The drawing under review shows one solid part. Ordinate dimensions are in mm from its lowest x, y, z. A direction names the side the tool comes from. Coordinates: 2 decimals unless noted, no trailing zeros. Order: outer loops, then holes, each group sorted by start corner. A loop starts at its lowest first (then second) coordinate and runs counter-clockwise, first axis right, second up.
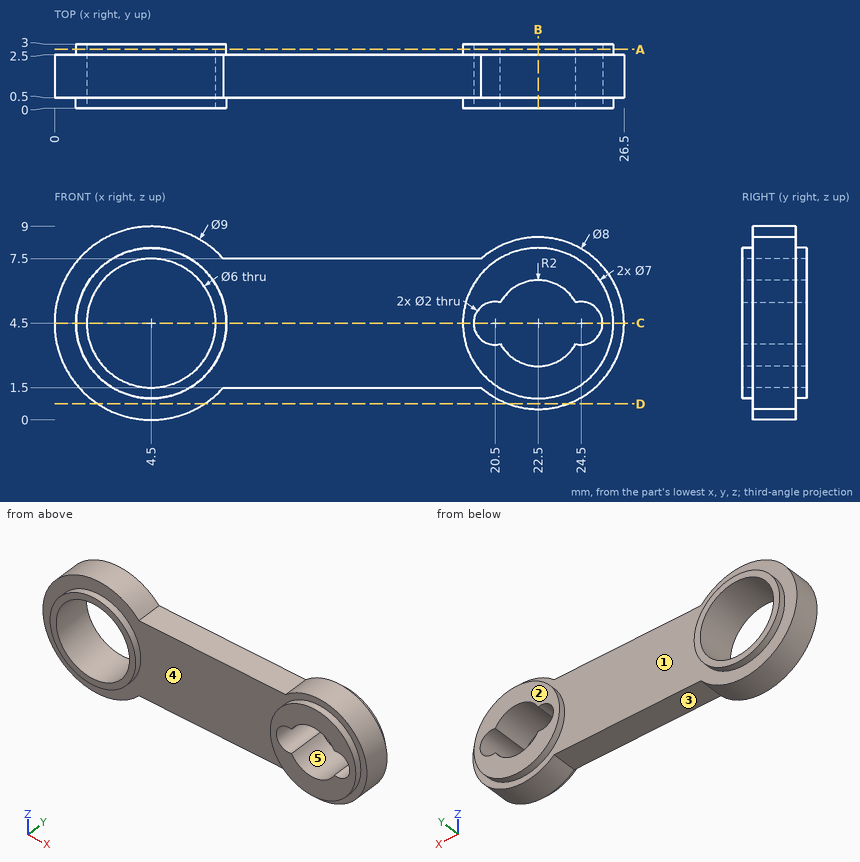
(1) We need section D-D, the plane z = 0.75. Write out the cut boundary in (x, y), and give its area (3 significant figures).
A:
outline: (2.01, 0.5) - (6.99, 0.5) - (6.99, 2.5) - (2.01, 2.5) - close; (21.11, 0.5) - (23.89, 0.5) - (23.89, 2.5) - (21.11, 2.5) - close
area: 15.5 mm2
(2) Wall thickness on probe 1 along X at (y, z) = (1.5, 4.5); probe 2 along Z at (x, y) = (4.5, 1.8); probe 3 along X at (y, z) = (1.95, 2.75): over which ranges is each line inside the solid? List them lowest first.
A:
probe 1: x = 0 to 1.5, 7.5 to 19.5, 25.5 to 26.5
probe 2: z = 0 to 1.5, 7.5 to 9
probe 3: x = 0.35 to 2.06, 6.94 to 21.53, 23.47 to 26.1
(3) We need section C-C, the plane z = 4.5. Write out the cut boundary in (x, y).
A:
outline: (0, 0.5) - (1, 0.5) - (1, 0) - (1.5, 0) - (1.5, 3) - (1, 3) - (1, 2.5) - (0, 2.5) - close; (7.5, 0) - (8, 0) - (8, 0.5) - (19, 0.5) - (19, 0) - (19.5, 0) - (19.5, 3) - (19, 3) - (19, 2.5) - (8, 2.5) - (8, 3) - (7.5, 3) - close; (25.5, 0) - (26, 0) - (26, 0.5) - (26.5, 0.5) - (26.5, 2.5) - (26, 2.5) - (26, 3) - (25.5, 3) - close
(4) We need section A-A, the plane y = 2.75. Write out the cut boundary in (x, z), and give its area (3 significant figures).
A:
outline: circle Ø7 at (4.5, 4.5); circle Ø7 at (22.5, 4.5); hole circle Ø6 at (4.5, 4.5); hole (20.75, 3.53) arc R2 ccw to (24.25, 3.53) arc R1 ccw (long way) to (24.25, 5.47) arc R2 ccw to (20.75, 5.47) arc R1 ccw (long way) to start
area: 32.7 mm2
(5) We need section B-B, the plane x = 22.5. Write out the cut boundary in (y, z).
A:
outline: (0, 1) - (0.5, 1) - (0.5, 0.5) - (2.5, 0.5) - (2.5, 1) - (3, 1) - (3, 2.5) - (0, 2.5) - close; (0, 6.5) - (3, 6.5) - (3, 8) - (2.5, 8) - (2.5, 8.5) - (0.5, 8.5) - (0.5, 8) - (0, 8) - close
(6) Machinability: for the marked faces 3, 4 and 5, which of the approach directions +Z, -Z, +X, -X, +Y, -Y give a long, thin tool a straight path to every point of the face, cutting with its end or side? Answer none if there is none.
A:
face 3: -Z, +Y, -Y
face 4: -Y
face 5: +Y, -Y
(7) For pin 1 Ø1.5 at (x, z) = (22.5, 4) entering from -Y; pin 2 Ø1.5 at (x, z) = (14, 2) entering from +Y; pin 3 Ø1 at (x, y) = (15, 1) entering from +Z; pin 4 Ø1 at (x, y) = (16, 1.5) entering from -Z, all flat-tipped, find the tip position at first contact; note any pin that passes through.
A:
pin 1: passes through
pin 2: stops at y = 2.5
pin 3: stops at z = 7.5
pin 4: stops at z = 1.5
(8) Draft analysis for pull direction X (two halves, no side actions). For the marked faces 1 and 2, state which applies: released by +X, released by -X, zero draft, split by the parting line, or undercut.
A:
face 1: undercut
face 2: zero draft
